```python
from build123d import *

# Parameters (mm, degrees)
F0_R     = 18.796
F2_DEPTH = 76.2
F1_R     = 6.35
F3_DEPTH = 127
F4_R     = 1.27
F5_W     = 2.54
F5_H     = 2.54
F6_DEPTH = 127
F7_R     = 2.54


with BuildPart() as f2:
    # F0 (on Front) → F2 (new body)
    with BuildSketch(Plane.XZ):
        Circle(F0_R)
    extrude(amount=F2_DEPTH)

    # F1 (on face) → F3 (join)
    with BuildSketch(Plane.XZ):
        Circle(F1_R)
    extrude(amount=F3_DEPTH)

    # F4
    f4_edges = [f2.edges().sort_by_distance(p)[0] for p in [
        (-18.796, 0, 0),
        (-6.35, -127, 0),
    ]]
    fillet(f4_edges, radius=F4_R)

    # F5 (on face) → F6 (cut)
    with BuildSketch(Plane.XZ.offset(127)):
        Rectangle(F5_W, F5_H)
    extrude(amount=-F6_DEPTH, mode=Mode.SUBTRACT)

    # F7
    f7_edges = [f2.edges().sort_by_distance(p)[0] for p in [
        (-18.796, -76.2, 0),
    ]]
    fillet(f7_edges, radius=F7_R)


solid = f2.part
```
Can you work these out from the model? Positions are in its coordinate system, mm. A direction names the side the tool comes from. Give positions to 0.01 mm unless a question says otherwise; leave off trailing zeros. Write each loop counter-clockwise with the first axis right and the second up, starting at its lowest first coordinate (ties: lowest second). Pieces come first, ordered by that corner, then holes. Notation, with made-up numbers: (61.5, -17.75) - (100.5, -17.75) arc R12 cw to (100.5, -11.75) - close; hole circle Ø2 at (-29, -16.75). An arc over 180 degrees is marked (long way). Write item = value, one per line. Start each with the question number.
1. Imagine slicing it at A-A (x = 0). Please give me the cut outline in (y, z).
2. Imagine slicing it at B-B (z = 0). Please give me the cut outline in (x, y), and give its area (3 significant figures).
3. On a 3-axis mill with a long thin cutter (end or side, diameter ignored), from which of +Z, -Z, +X, -X, +Y, -Y can I reach the whole of each face in a straight line? I mean faces 5 (the face through (4, 0, 0)), 6 (the face through (0, -64, 1.27)). Say none if no direction works.
4. Please list where these lines run through material, in increasing order: line 1 (X direction, y = -9, z = -0.5); line 2 (Y direction, x = 7.5, z = -13); line 3 (Z direction, x = 9.5, y = -46).
5. Thinking about a two-plate mould opening in Z: for faces 1 (the face through (1.27, -64, 0)), 2 (the face through (-1.27, -64, 0)), 3 (the face through (-1.38, -100.62, -6.2)), 4 (the face through (7, -76.2, 0)), which applies, released by +Z, released by -Z, zero draft, split by the parting line, or undercut?
6. For pin 1 (3 mm diameter, centred on y = -90.5, z = -1.5, fed in from +X); pin 2 (5 mm diameter, centred on y = -89.5, z = -8, fed in from -X); pin 3 (0.8 mm diameter, centred on x = 0, y = -84, fed in from -Z), each with a flat end and sliding along its axis, tell me the tip position at first contact or that it passes through.
7. Imagine slicing it at C-C (y = -112.5). Please give me the cut outline in (x, z), and give its area (3 significant figures).
8. Imagine slicing it at D-D (y = -62.5). Please give me the cut outline in (x, z), and give its area (3 significant figures).
Worked answers:
q1.outline = (-127, -5.08) arc R1.27 ccw to (-125.73, -6.35) - (-76.2, -6.35) - (-76.2, -16.26) arc R2.54 ccw to (-73.66, -18.8) - (-1.27, -18.8) arc R1.27 ccw to (0, -17.53) - (0, -1.27) - (-127, -1.27) - close; (-127, 1.27) - (0, 1.27) - (0, 17.53) arc R1.27 ccw to (-1.27, 18.8) - (-73.66, 18.8) arc R2.54 ccw to (-76.2, 16.26) - (-76.2, 6.35) - (-125.73, 6.35) arc R1.27 ccw to (-127, 5.08) - close
q2.outline = (-18.8, -73.66) arc R2.54 ccw to (-16.26, -76.2) - (-6.35, -76.2) - (-6.35, -125.73) arc R1.27 ccw to (-5.08, -127) - (-1.27, -127) - (-1.27, 0) - (-17.53, 0) arc R1.27 ccw to (-18.8, -1.27) - close; (1.27, -127) - (5.08, -127) arc R1.27 ccw to (6.35, -125.73) - (6.35, -76.2) - (16.26, -76.2) arc R2.54 ccw to (18.8, -73.66) - (18.8, -1.27) arc R1.27 ccw to (17.53, 0) - (1.27, 0) - close
q2.area = 3,180 mm2
q3.face_5 = +Z, -Z, +X, -X, +Y
q3.face_6 = +Y, -Y
q4.line_1 = -18.79 to -1.27, 1.27 to 18.79
q4.line_2 = -76.2 to 0
q4.line_3 = -16.22 to 16.22
q5.face_1 = undercut
q5.face_2 = undercut
q5.face_3 = split by the parting line
q5.face_4 = zero draft
q6.pin_1 = 6.35
q6.pin_2 = -3.17
q6.pin_3 = -6.35
q7.outline = circle Ø12.7 at (0, 0); hole (-1.27, -1.27) - (1.27, -1.27) - (1.27, 1.27) - (-1.27, 1.27) - close
q7.area = 120 mm2
q8.outline = circle Ø37.59 at (0, 0); hole (-1.27, -1.27) - (1.27, -1.27) - (1.27, 1.27) - (-1.27, 1.27) - close
q8.area = 1,100 mm2
